Verification items for the finished model (mm, model axes). Give positions to 0.01 mm unless a question says otherwise; leave off trailing zeros. Write each loop counter-clockwise with the first axis right and the second up, starting at its lowest first coordinate (ties: lowest second). Pieces come first, ordered by that corner, then holes. Notation, with made-up numbers: (9, 86.5) - (36, 86.5) arc R26 ccw to (36, 100.5) - close; hole circle Ø1 at (89, -2.75). An arc over 180 degrees is marked (long way). Answer as a JSON object with one key per item and string values. Group by question number.
Item 1: Sectioned sample at C-C, the plane y = 0. Record the boundary of the cut face in (x, z).
Item 2: Sectioned sample at A-A, the plane z = 0.7. Record the boundary of the cut face in (x, y) (3 decimals), and give its area (3 significant figures).
Item 3: Sectioned sample at D-D, the plane y = 39. Record the boundary of the cut face in (x, z) (3 decimals), and give its area (3 significant figures).
Item 4: Go/stop test with flat-tipped pins: pin 1 (0.5 mm diameter, centred on y = -29.5, z = 0.5, fed in from +X); pin 2 (19.5 mm diameter, centred on x = -47, y = -52, fed in from +Z). Record where each tip stops, or that it passes through.
Item 5: Scan lines: line 1 along Y through (x, z) = (-48, 0.5); line 2 along X through (y, z) = (35.5, 0.8) (3 decimals); line 3 along Y through (x, z) = (47.5, 0.55). Record each from-to range of solid material in increasing order. Write a range as [from, to].
Item 6: Sectioned sample at B-B, the plane x = 0. Record the boundary of the cut face in (y, z), and give its area (3 significant figures).
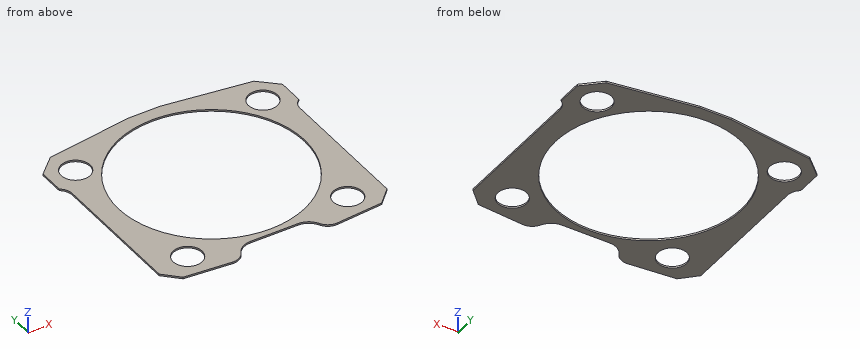
```python
from build123d import *

# Parameters (mm, degrees)
SKETCH1_R           = 54.5
SKETCH1_R_2         = 8.5
BOSS_EXTRUDE1_DEPTH = 1


with BuildPart() as part:
    # Sketch1 → Boss-Extrude1 (new body)
    with BuildSketch(Plane.XY):
        with BuildLine():
            Line((-9.25, 62), (9.25, 62))
            Line((9.25, 62), (59.753671506, 54.902171851))
            Line((59.753671506, 54.902171851), (70.375, 44.997622795))
            Line((70.375, 44.997622795), (70.375, 30))
            ThreePointArc((70.375, 30), (67.821864652, 27.130969792), (66.9, 23.402699416))
            Line((66.9, 23.402699416), (66.9, -57))
            Line((66.9, -57), (58.333823358, -65.566176642))
            Line((58.333823358, -65.566176642), (30.863053479, -67.969557585))
            ThreePointArc((30.863053479, -67.969557585), (26.471818631, -67.096086665), (23.237604307, -64))
            Line((23.237604307, -64), (22.660254038, -63))
            ThreePointArc((22.660254038, -63), (19, -59.339745962), (14, -58))
            Line((14, -58), (-14, -58))
            ThreePointArc((-14, -58), (-19, -59.339745962), (-22.660254038, -63))
            Line((-22.660254038, -63), (-23.237604307, -64))
            ThreePointArc((-23.237604307, -64), (-26.471818631, -67.096086665), (-30.863053479, -67.969557585))
            Line((-30.863053479, -67.969557585), (-58.333823358, -65.566176642))
            Line((-58.333823358, -65.566176642), (-66.9, -57))
            Line((-66.9, -57), (-66.9, 23.402699416))
            ThreePointArc((-66.9, 23.402699416), (-67.821864652, 27.130969792), (-70.375, 30))
            Line((-70.375, 30), (-70.375, 44.997622795))
            Line((-70.375, 44.997622795), (-59.753671506, 54.902171851))
            Line((-59.753671506, 54.902171851), (-9.25, 62))
        make_face()
        Circle(SKETCH1_R, mode=Mode.SUBTRACT)
        with Locations((55, 39)):
            Circle(SKETCH1_R_2, mode=Mode.SUBTRACT)
        with Locations(Location((-55, 39, 0), (0, 0, 180))):
            Circle(SKETCH1_R_2, mode=Mode.SUBTRACT)
        with Locations((47, -52)):
            Circle(SKETCH1_R_2, mode=Mode.SUBTRACT)
        with Locations(Location((-47, -52, 0), (0, 0, 180))):
            Circle(SKETCH1_R_2, mode=Mode.SUBTRACT)
    extrude(amount=BOSS_EXTRUDE1_DEPTH)


solid = part.part
```
Geometry check:
{
 "1": {"outline": "(-66.9, 0) - (-54.5, 0) - (-54.5, 1) - (-66.9, 1) - close; (54.5, 0) - (66.9, 0) - (66.9, 1) - (54.5, 1) - close"},
 "2": {"outline": "(-70.375, 30) arc R8 cw to (-66.9, 23.403) - (-66.9, -57) - (-58.334, -65.566) - (-30.863, -67.97) arc R8 ccw to (-23.238, -64) - (-22.66, -63) arc R10 cw to (-14, -58) - (14, -58) arc R10 cw to (22.66, -63) - (23.238, -64) arc R8 ccw to (30.863, -67.97) - (58.334, -65.566) - (66.9, -57) - (66.9, 23.403) arc R8 cw to (70.375, 30) - (70.375, 44.998) - (59.754, 54.902) - (9.25, 62) - (-9.25, 62) - (-59.754, 54.902) - (-70.375, 44.998) - close; hole circle Ø17 at (-55, 39); hole circle Ø17 at (-47, -52); hole circle Ø109 at (0, 0); hole circle Ø17 at (47, -52); hole circle Ø17 at (55, 39)", "area": "6,140 mm^2"},
 "3": {"outline": "(-70.375, 0) - (-63.5, 0) - (-63.5, 1) - (-70.375, 1) - close; (-46.5, 0) - (-38.069, 0) - (-38.069, 1) - (-46.5, 1) - close; (38.069, 0) - (46.5, 0) - (46.5, 1) - (38.069, 1) - close; (63.5, 0) - (70.375, 0) - (70.375, 1) - (63.5, 1) - close", "area": "30.6 mm^2"},
 "4": {"pin 1": "x = 66.9", "pin 2": "z = 1"},
 "5": {"line 1": "[-66.47, -60.44], [-43.56, -25.81], [25.81, 34.18], [43.82, 56.55]", "line 2": "[-70.375, -62.746], [-47.254, -41.352], [41.352, 47.254], [62.746, 70.375]", "line 3": "[-66.51, -60.49], [-43.51, -26.72], [26.72, 35], [43, 56.62]"},
 "6": {"outline": "(-58, 0) - (-54.5, 0) - (-54.5, 1) - (-58, 1) - close; (54.5, 0) - (62, 0) - (62, 1) - (54.5, 1) - close", "area": "11.0 mm^2"}
}
